```python
from build123d import *

# Parameters (mm, degrees)
ESBO_O1_W                     = 32
ESBO_O1_H                     = 17
RESSALTO_EXTRUS_O1_DEPTH      = 15
RESSALTO_EXTRUS_O2_DEPTH      = 45
RESSALTO_EXTRUS_O2_DEPTH_BACK = 3
ESBO_O2_W                     = 6
ESBO_O2_H                     = 15
ESBO_O3_W                     = 40
ESBO_O3_H                     = 15
RESSALTO_EXTRUS_O3_DEPTH      = 3
CORTE_EXTRUS_O1_DEPTH         = 84.736797348
CORTE_EXTRUS_O1_DEPTH_BACK    = 6
ESBO_O5_R                     = 2.45
CORTE_EXTRUS_O2_DEPTH         = 12
CORTE_EXTRUS_O3_DEPTH         = 72.02091848
CORTE_EXTRUS_O3_DEPTH_BACK    = 72.02091848
ESBO_O8_R                     = 1
CORTE_EXTRUS_O4_DEPTH         = 72.588901806
CORTE_EXTRUS_O4_DEPTH_BACK    = 72.588901806
ESBO_O9_W                     = 20.5
ESBO_O9_H                     = 9


with BuildPart() as part:
    # Esboço1 → Ressalto-extrusão1 (new body)
    with BuildSketch(Plane.XY):
        with Locations((-30.614733331, -8.145893332)):
            Rectangle(ESBO_O1_W, ESBO_O1_H)
    extrude(amount=RESSALTO_EXTRUS_O1_DEPTH)

    # Esboço2 → Ressalto-extrusão2 (add, two sides: drawn at the far end of the back side and taken through both)
    with BuildSketch(Plane(origin=(0, 0.354106668, 0), x_dir=(1, 0, 0), z_dir=(0, 1, 0)).offset(-RESSALTO_EXTRUS_O2_DEPTH_BACK)):
        with Locations((-30.614733331, -7.5)):
            Rectangle(ESBO_O2_W, ESBO_O2_H)
    extrude(amount=RESSALTO_EXTRUS_O2_DEPTH + RESSALTO_EXTRUS_O2_DEPTH_BACK)

    # Esboço3 → Ressalto-extrusão3 (add)
    with BuildSketch(Plane(origin=(0, 45.354106668, 0), x_dir=(1, 0, 0), z_dir=(0, 1, 0))):
        with Locations((-30.614733331, -7.5)):
            Rectangle(ESBO_O3_W, ESBO_O3_H)
    extrude(amount=RESSALTO_EXTRUS_O3_DEPTH)

    # Esboço5 → Corte-extrusão1 (cut, two sides: drawn at the far end of the back side and taken through both)
    with BuildSketch(Plane(origin=(0, 48.354106668, 0), x_dir=(1, 0, 0), z_dir=(0, 1, 0)).offset(-CORTE_EXTRUS_O1_DEPTH_BACK)):
        with Locations(Location((-46.614733331, -4, 0), (0, 0, 90))):
            Circle(ESBO_O5_R)
        with Locations(Location((-14.614733331, -11, 0), (0, 0, 90))):
            Circle(ESBO_O5_R)
    extrude(amount=CORTE_EXTRUS_O1_DEPTH + CORTE_EXTRUS_O1_DEPTH_BACK, mode=Mode.SUBTRACT)

    # Esboço7 → Corte-extrusão2 (cut)
    with BuildSketch(Plane.XY.offset(15)):
        Polygon((-44.914733331, -15.645893332), (-44.914733331, -0.645893332), (-32.972451845, -0.645893332), (-32.972451845, -3.645893332), (-16.314733331, -3.645893332), (-16.314733331, -15.645893332), align=None)
    extrude(amount=-CORTE_EXTRUS_O2_DEPTH, mode=Mode.SUBTRACT)

    # Esboço8 → Corte-extrusão3 (cut, two sides: drawn at the far end of the back side and taken through both)
    with BuildSketch(Plane.XY.offset(3).offset(-CORTE_EXTRUS_O3_DEPTH_BACK)):
        with Locations((-42.364733331, -13.395893332)):
            Circle(ESBO_O8_R)
        with Locations((-18.864733331, -5.895893332)):
            Circle(ESBO_O8_R)
    extrude(amount=CORTE_EXTRUS_O3_DEPTH + CORTE_EXTRUS_O3_DEPTH_BACK, mode=Mode.SUBTRACT)

    # Esboço9 → Corte-extrusão4 (cut, two sides: drawn at the far end of the back side and taken through both)
    with BuildSketch(Plane(origin=(0, 0, 0), x_dir=(-1, 0, 0), z_dir=(0, 0, -1)).offset(-CORTE_EXTRUS_O4_DEPTH_BACK)):
        with Locations((30.614733331, -9.645893332)):
            Rectangle(ESBO_O9_W, ESBO_O9_H)
    extrude(amount=CORTE_EXTRUS_O4_DEPTH + CORTE_EXTRUS_O4_DEPTH_BACK, mode=Mode.SUBTRACT)


solid = part.part
```
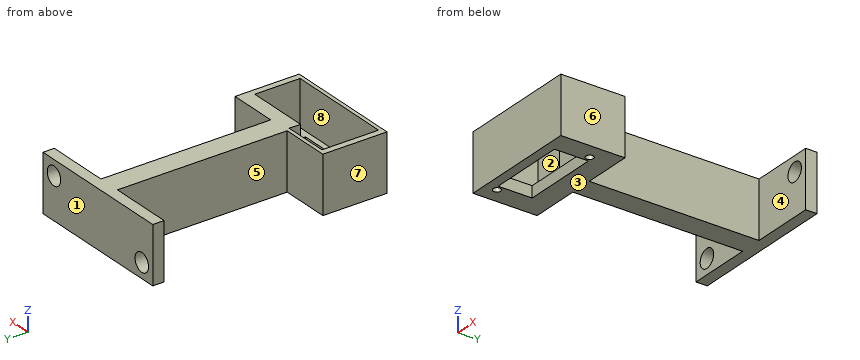
Design review of the part built by this model. Coordinates are the model's own, in mm. Face numbers are marked on the shaded views. A direction names the side the tool comes from. Coordinates: 2 decimals unless noted, no trailing zeros. Order: outer loops, then holes, each group sorted by start corner. A loop starts at its lowest first (then second) coordinate and runs counter-clockwise, first axis right, second up. Notation, with made-up numbers: (-2, -6) - (4, -6) arc R23 ccw to (4, 2) - close; hole circle Ø4 at (48, 39). An arc over 180 degrees is marked (long way). Answer in a Markdown table with one row per item.
(1) The part is to be moulded in two halves that separate along Y. For the marked faces 1, 2 and 3, say which applies: released by +Y, released by -Y, zero draft, split by the parting line, or undercut.
Checked values:
| item | result |
|---|---|
| face 1 | released by +Y |
| face 2 | undercut |
| face 3 | zero draft |
(2) Consider section A-A on x = -39.5. State the section outline as (y, z) points.
Checked values:
| item | result |
|---|---|
| outline | (-16.65, 0) - (-14.15, 0) - (-14.15, 3) - (-15.65, 3) - (-15.65, 15) - (-16.65, 15) - close; (-5.15, 0) - (0.35, 0) - (0.35, 15) - (-0.65, 15) - (-0.65, 3) - (-5.15, 3) - close; (45.35, 0) - (48.35, 0) - (48.35, 15) - (45.35, 15) - close |
(3) Consider section B-B on z = 11. State the section outline as (x, y) points.
Checked values:
| item | result |
|---|---|
| outline | (-50.61, 45.35) - (-33.61, 45.35) - (-33.61, 0.35) - (-46.61, 0.35) - (-46.61, -16.65) - (-14.61, -16.65) - (-14.61, 0.35) - (-27.61, 0.35) - (-27.61, 45.35) - (-17.06, 45.35) - (-17.06, 48.35) - (-50.61, 48.35) - close; (-12.16, 45.35) - (-10.61, 45.35) - (-10.61, 48.35) - (-12.16, 48.35) - close; hole (-44.91, -15.65) - (-16.31, -15.65) - (-16.31, -3.65) - (-32.97, -3.65) - (-32.97, -0.65) - (-44.91, -0.65) - close |
(4) For the marked faces 4, 5, 6, 7 and 8, list the 3-axis set-ups (+Z, -Z, +X, -X, +Y, -Y) from which the entire face can be reached by the end or side of a thin tool; tool diameter is ignored.
Checked values:
| item | result |
|---|---|
| face 4 | +Z, -Z, +X |
| face 5 | +Z, -Z, -X |
| face 6 | +Z, -Z, +X, -Y |
| face 7 | +Z, -Z, -X, -Y |
| face 8 | +Z |
(5) Consider section D-D on z = 7.75. State the section outline as (x, y) points, plus the area to 3 significant figures.
Checked values:
| item | result |
|---|---|
| outline | (-50.61, 45.35) - (-33.61, 45.35) - (-33.61, 0.35) - (-46.61, 0.35) - (-46.61, -16.65) - (-14.61, -16.65) - (-14.61, 0.35) - (-27.61, 0.35) - (-27.61, 45.35) - (-10.61, 45.35) - (-10.61, 48.35) - (-50.61, 48.35) - close; hole (-44.91, -15.65) - (-16.31, -15.65) - (-16.31, -3.65) - (-32.97, -3.65) - (-32.97, -0.65) - (-44.91, -0.65) - close |
| area | 555 mm^2 |
(6) Consider section C-C on x = -29. State the section outline as (y, z) points, plus the area to 3 significant figures.
Checked values:
| item | result |
|---|---|
| outline | (-16.65, 0) - (-14.15, 0) - (-14.15, 3) - (-15.65, 3) - (-15.65, 15) - (-16.65, 15) - close; (-5.15, 0) - (48.35, 0) - (48.35, 15) - (-3.65, 15) - (-3.65, 3) - (-5.15, 3) - close |
| area | 804 mm^2 |
(7) Wall thickness on line 1 along Y through (x, z) = (-27, 8.75); line 2 along Y through (x, z) = (-44, 7); line 3 along Y through (x, z) = (-41, 1.5): over which ranges is each line inside the solid? List them lowest first. Write a range as from..to.
Checked values:
| item | result |
|---|---|
| line 1 | -16.65..-15.65, -3.65..0.35, 45.35..48.35 |
| line 2 | -16.65..-15.65, -0.65..0.35, 45.35..48.35 |
| line 3 | -16.65..0.35, 45.35..48.35 |
(8) Clearance check with flat-ended pins moving along their axes: pin 1 (5 mm diameter, centred on y = 24.5, z = 6.5, fed in from +X); pin 2 (2.5 mm diameter, centred on y = -1.5, z = 10, fed in from -X); pin 3 (1.6 mm diameter, centred on x = -18.86, y = -5.9, fed in from -Z); pin 4 (3 mm diameter, centred on x = -14.61, z = 11, fed in from +Y). State where each tip first meets the part, or that it passes through.
Checked values:
| item | result |
|---|---|
| pin 1 | x = -27.61 |
| pin 2 | x = -46.61 |
| pin 3 | through |
| pin 4 | y = 0.35 |
